from build123d import *

# Parameters (mm, degrees)
F0_R     = 6
F1_DEPTH = 15
F3_DEPTH = 5
F5_DEPTH = 3
F6_R     = 9.527798
F6_R_2   = 7.870818
F7_DEPTH = 3


with BuildPart() as f1:
    # F0 (on Top) → F1 (new body)
    with BuildSketch(Plane.XY):
        Circle(F0_R)
    extrude(amount=F1_DEPTH)

    # F2 (on face) → F3 (cut)
    with BuildSketch(Plane.XY.offset(15)):
        Polygon((1.911385, 1.911385), (0, 2.703106), (-1.911385, 1.911385), (-2.703106, 0), (-1.911385, -1.911385), (0, -2.703106), (1.911385, -1.911385), (2.703106, 0), align=None)
    extrude(amount=-F3_DEPTH, mode=Mode.SUBTRACT)

    # F4 (on face) → F5 (join)
    with BuildSketch(Plane(origin=(0, 0, 0), x_dir=(1, 0, 0), z_dir=(0, 0, -1))):
        Polygon((-6.211701, -11.975178), (13.476659, 0.608098), (-7.264957, 11.36708), align=None)
    extrude(amount=F5_DEPTH)

    # F6 (on face) → F7 (join)
    with BuildSketch(Plane(origin=(0, 0, -3), x_dir=(1, 0, 0), z_dir=(0, 0, -1))):
        Circle(F6_R)
        Circle(F6_R_2, mode=Mode.SUBTRACT)
    extrude(amount=-F7_DEPTH)


solid = f1.part
Check sheet for the modelled part. Datum: model origin and axes. Units: mm. A direction names the side the tool comes from. Round coordinates to 2 decimals unless told otherwise and drop trailing zeros. Order: outer loops, then holes, each group sorted by start corner. A loop starts at its lowest first (then second) coordinate and runs counter-clockwise, first axis right, second up.
(1) Scan lines: probe 1 along Y at (x, z) = (0.75, -1.25) (3 decimals); probe 2 along Z at (x, y) = (-4.75, 8.25); probe 3 along X at (y, z) = (5, -1.25). Record each from-to range of solid material in increasing order.
(2) Cross-section at D-D, the plane x = -5.25. Enter the section's corners in (y, z).
(3) Draft check along Y on faces 1 (the flat face through (-4.154, 10.66, -1.479)), 2 (the flat face through (11.31, -1.73, -1.48)), 3 (the flat face through (0, 0, 10)), 4 (the flat face through (4, -5, 0)). Enter one of: pulls with the +Y half, pulls with the -Y half, needs draft (parallel to the pull), parting line crosses it, or undercut.
(4) Cross-section at C-C, the plane x = 3.75. Enter the section's corners in (y, z).
(5) Cross-section at B-B, the plane y = -7. Enter the section's corners in (x, z), and give its area (3 significant figures).
(6) Access from +Z, -Z, +X, -X, +Y, -Y to the whole of each face (thin tool, end or side, straight path). Record for faces 5 (the flat face through (3.16, -5.96, -1.48)), 6 (the flat face through (-2.313, -0.942, 12.535)), 7 (the flat face through (-7.155, -8.927, -1.479)).
(7) Go/stop test with flat-tipped pins: P1, Ø8, axis at y = -8.5, z = 7.5, coming from the -X side; P2, Ø4, axis at y = -1.5, z = 5.5, coming from the -X side; P3, Ø1, axis at y = -1.5, z = 6.5, coming from the +X side. Record where each tip stops, or that it passes through.
(8) Cross-section at A-A, the plane z = 13.5. Enter the section's corners in (x, y), and give its area (3 significant figures).
Check sheet entries:
1. probe 1: y = -9.498 to -7.835, -7.21 to 7.526, 7.835 to 9.498
1. probe 2: z = -3 to 0
1. probe 3: x = -8.11 to 4.7, 6.08 to 8.11
2. outline: (-10.32, -3) - (11.36, -3) - (11.36, 0) - (2.9, 0) - (2.9, 15) - (-2.9, 15) - (-2.9, 0) - (-10.32, 0) - close
3. face 1: pulls with the +Y half
3. face 2: pulls with the -Y half
3. face 3: undercut
3. face 4: needs draft
4. outline: (-8.76, -3) - (-6.92, -3) - (-6.92, 0) - (-8.76, 0) - close; (-5.65, -3) - (5.61, -3) - (5.61, 0) - (4.68, 0) - (4.68, 15) - (-4.68, 15) - (-4.68, 0) - (-5.65, 0) - close; (6.92, -3) - (8.76, -3) - (8.76, 0) - (6.92, 0) - close
5. outline: (-7.07, -3) - (1.15, -3) - (1.15, 0) - (-7.07, 0) - close; (3.6, -3) - (6.46, -3) - (6.46, 0) - (3.6, 0) - close
5. area: 33.3 mm2
6. face 5: +Z, -Z
6. face 6: +Z
6. face 7: +Z, -Z, -X
7. P1: stops at x = -3.97
7. P2: stops at x = -6
7. P3: stops at x = 5.92
8. outline: circle Ø12 at (0, 0); hole (-2.7, 0) - (-1.91, -1.91) - (0, -2.7) - (1.91, -1.91) - (2.7, 0) - (1.91, 1.91) - (0, 2.7) - (-1.91, 1.91) - close
8. area: 92.4 mm2
